Can you work these out from the model? Positions are in its coordinate system, mm. Round coordinates to 2 decimals unless told otherwise and drop trailing zeros. Write each loop counter-clockwise with the first axis right and the second up, starting at its lowest first coordinate (ties: lowest second). Pieces come first, ordered by that corner, then holes.
Q1. If we section it at B-B (z = 1.8): Give the number of separate pieces and of enclosed holes in the cut face, plus the area to 3 significant figures.
Q2. We'd pull the mould along X, two halves only. Please class faces 1 (the cylindrical face through (-51.81, 23.177, 1.479)), 2 (the flat face through (-79.233, 62, 1)), 3 (the flat face through (-19.09, 112.21, 1.48)), 4 (the flat face through (-44, 122.351, 1)): +X half, -X half, draft (parallel to the pull), parting line (faces both ways), or undercut.
Q3. If we section it at C-C (x = -66): Please give me the cut outline in (y, z), plus the area to 3 significant figures.
Q4. If we section it at D-D (y = 111.5): Please give me the cut outline in (x, z).
Q5. If we section it at A-A (x = -51): Please give me the cut outline in (y, z).
Q6. I'm going to push a flat-ended pin straight in: pin 1 Ø2 at (x, y) = (-37.23, 104.29) entering from +Z. Where does the tip first touch, or does it pass through?
Q7. Please list where these lines run through material, in increasing order: line 1 along X through (y, z) = (72.5, 1.55); line 2 along X through (y, z) = (71, 0.85); line 3 along Y through (x, z) = (-14, 1.65).
from build123d import *

# Parameters (mm, degrees)
SKETCH_1_W          = 70
SKETCH_1_H          = 100
EXTRUDE_1_DEPTH     = 3
SKETCH_2_R          = 1.6
CUT_EXTRUDE_1_DEPTH = 3
SKETCH_3_R          = 1.25
CUT_EXTRUDE_2_DEPTH = 3
CHAMFER_1_SIZE      = 20


with BuildPart() as part:
    # 草图1 → 凸台-拉伸1 (new body)
    with BuildSketch(Plane.XY):
        with Locations((-44.233232324, 72.350653578)):
            Rectangle(SKETCH_1_W, SKETCH_1_H)
    extrude(amount=EXTRUDE_1_DEPTH)

    # 草图2 → 切除-拉伸1 (cut)
    with BuildSketch(Plane.XY.offset(3)):
        with Locations((-74.233232324, 32.350653578)):
            Circle(SKETCH_2_R)
        with Locations((-14.233232324, 32.350653578)):
            Circle(SKETCH_2_R)
        with Locations((-14.233232324, 72.286219849)):
            Circle(SKETCH_2_R)
        with Locations((-74.233232324, 72.286219849)):
            Circle(SKETCH_2_R)
    extrude(amount=-CUT_EXTRUDE_1_DEPTH, mode=Mode.SUBTRACT)

    # 草图3 → 切除-拉伸2 (cut)
    with BuildSketch(Plane(origin=(0, 0, 0), x_dir=(-1, 0, 0), z_dir=(0, 0, -1))):
        with Locations((37.233066324, 104.286219849)):
            Circle(SKETCH_3_R)
        with Locations((51.233066324, 104.286219849)):
            Circle(SKETCH_3_R)
        with Locations((37.233066324, 24.286219849)):
            Circle(SKETCH_3_R)
        with Locations((51.233066324, 24.286219849)):
            Circle(SKETCH_3_R)
        with Locations((34.233232324, 121.536231848)):
            Circle(SKETCH_3_R)
        with Locations((54.233232324, 121.536231848)):
            Circle(SKETCH_3_R)
    extrude(amount=-CUT_EXTRUDE_2_DEPTH, mode=Mode.SUBTRACT)

    # 倒角1
    chamfer_1_edges = [part.edges().sort_by_distance(p)[0] for p in [
        (-79.233232324, 122.350653578, 1.5),
        (-9.233232324, 122.350653578, 1.5),
    ]]
    chamfer(chamfer_1_edges, length=CHAMFER_1_SIZE)


solid = part.part
A:
1. separate pieces: 1
1. enclosed holes: 8
1. area: 6,540 mm2
2. face 1: undercut
2. face 2: -X half
2. face 3: +X half
2. face 4: draft
3. outline: (22.35, 0) - (115.58, 0) - (115.58, 3) - (22.35, 3) - close
3. area: 280 mm2
4. outline: (-70.08, 0) - (-18.38, 0) - (-18.38, 3) - (-70.08, 3) - close
5. outline: (22.35, 0) - (23.06, 0) - (23.06, 3) - (22.35, 3) - close; (25.51, 0) - (103.06, 0) - (103.06, 3) - (25.51, 3) - close; (105.51, 0) - (122.35, 0) - (122.35, 3) - (105.51, 3) - close
6. pin 1: passes through
7. line 1: x = -79.23 to -75.82, -72.65 to -15.82, -12.65 to -9.23
7. line 2: x = -79.23 to -75.18, -73.28 to -15.18, -13.28 to -9.23
7. line 3: y = 22.35 to 30.77, 33.93 to 70.7, 73.87 to 107.12
